```python
from build123d import *

# Parameters (mm, degrees)
F0_R     = 3
F0_R_2   = 0.3
F1_DEPTH = 13
F0_R_3   = 3.3
F2_DEPTH = 6
F3_DEPTH = 6


with BuildPart() as f1:
    # F0 (on Front) → F1 (new body)
    with BuildSketch(Plane.XZ):
        Circle(F0_R)
        with Locations((0, -0.5961988354)):
            Circle(F0_R_2, mode=Mode.SUBTRACT)
        with Locations((0, 0.7511804579)):
            Circle(F0_R_2, mode=Mode.SUBTRACT)
        with Locations((0, 0.7511804579)):
            Circle(F0_R_2)
        with Locations((0, -0.5961988354)):
            Circle(F0_R_2)
    extrude(amount=F1_DEPTH)

    # F0 (on Front) → F2 (join)
    with BuildSketch(Plane.XZ):
        Circle(F0_R_3)
        Circle(F0_R, mode=Mode.SUBTRACT)
    extrude(amount=F2_DEPTH)

    # F0 (on Front) → F3 (join)
    with BuildSketch(Plane.XZ):
        with Locations((0, 0.7511804579)):
            Circle(F0_R_2)
        with Locations((0, -0.5961988354)):
            Circle(F0_R_2)
    extrude(amount=-F3_DEPTH)


solid = f1.part
```
Verification items for the finished model (mm, model axes). A direction names the side the tool comes from. Coordinates: 2 decimals unless noted, no trailing zeros. Loops run counter-clockwise (first coordinate to the right, second up) from the corner with the lowest first, then second, coordinate; pieces in that order, holes last. Notation, with made-up numbers: (58, -2) -> (81, -2) arc R33 ccw to (81, 31) -> close; hole circle Ø4 at (-4, 26.25). An arc over 180 degrees is marked (long way). Answer in a Markdown table with one row per item. Add a question column.
1. Section check B-B, the plane z = 0. Enter the section's corners in (x, y).
2. Section check C-C, the plane y = -10.5. Enter the section's corners in (x, z), then the cut area to 3 significant figures.
3. Section check A-A, the plane x = 0. Enter the section's corners in (y, z), then the cut area to 3 significant figures.
4. Material ranges on probe 1 along Y at (x, z) = (-1, 0); probe 2 along Z at (x, y) = (0, -8); probe 3 along Z at (x, y) = (-2, -5.5), recorded low to high. Write a range as [from, to].
5. Section check D-D, the plane x = -2. Enter the section's corners in (y, z).
6. Access from +Z, -Z, +X, -X, +Y, -Y to the whole of each face (thin tool, end or side, straight path). Record for faces 1 (the face through (-3, -9, 0)), 2 (the face through (-2.43, -2.96, 2.23)).
Derived:
| question | item | result |
|---|---|---|
| 1 | outline | (-3.3, -6) -> (-3, -6) -> (-3, -13) -> (3, -13) -> (3, -6) -> (3.3, -6) -> (3.3, 0) -> (-3.3, 0) -> close |
| 2 | outline | circle Ø6 at (0, 0) |
| 2 | area | 28.3 mm² |
| 3 | outline | (-13, -3) -> (-6, -3) -> (-6, -3.3) -> (0, -3.3) -> (0, -0.9) -> (6, -0.9) -> (6, -0.3) -> (0, -0.3) -> (0, 0.45) -> (6, 0.45) -> (6, 1.05) -> (0, 1.05) -> (0, 3.3) -> (-6, 3.3) -> (-6, 3) -> (-13, 3) -> close |
| 3 | area | 88.8 mm² |
| 4 | probe 1 | y = [-13, 0] |
| 4 | probe 2 | z = [-3, 3] |
| 4 | probe 3 | z = [-2.62, 2.62] |
| 5 | outline | (-13, -2.24) -> (-6, -2.24) -> (-6, -2.62) -> (0, -2.62) -> (0, 2.62) -> (-6, 2.62) -> (-6, 2.24) -> (-13, 2.24) -> close |
| 6 | face 1 | -Y |
| 6 | face 2 | +Y, -Y |
